```python
from build123d import *

# Parameters (mm, degrees)
F0_R      = 12.5
F1_DEPTH  = 76
F2_W      = 38
F2_H      = 46
F3_DEPTH  = 177
F5_DEPTH  = 67
F6_DEPTH  = 65
F7_W      = 51.9999994738
F7_H      = 11
F8_DEPTH  = 54
F10_DEPTH = 64


with BuildPart() as f1:
    # F0 (on Front) → F1 (new body)
    with BuildSketch(Plane.XZ):
        Polygon((-120, -10.9966229647), (0, -10.9966229647), (0, 7.0033770353), (-56, 7.0033770353), (-56, 61.0033770353), (-120, 61.0033770353), align=None)
        with Locations((-88, 25.0033770353)):
            Circle(F0_R, mode=Mode.SUBTRACT)
    extrude(amount=-F1_DEPTH)

    # F2 (on face) → F3 (cut)
    with BuildSketch(Plane.XY.offset(61.0033770353)):
        with Locations((-88, 36)):
            Rectangle(F2_W, F2_H)
    extrude(amount=-F3_DEPTH, mode=Mode.SUBTRACT)

    # F4 (on face) → F5 (cut)
    with BuildSketch(Plane.XY.offset(7.0033770353)):
        with BuildLine():
            ThreePointArc((-36.0197160629, 75.9483659138), (-10.4386975125, 64.1605543748), (0, 38))
            Line((0, 38), (0, 76))
            Line((0, 76), (-36.0197160629, 75.9483659138))
        make_face()
    extrude(amount=-F5_DEPTH, mode=Mode.SUBTRACT)

    # F4 (on face) → F6 (cut)
    with BuildSketch(Plane.XY.offset(7.0033770353)):
        with BuildLine():
            ThreePointArc((-36.0197160629, 75.9483659138), (-10.4386975125, 64.1605543748), (0, 38))
            Line((0, 38), (0, 76))
            Line((0, 76), (-36.0197160629, 75.9483659138))
        make_face()
        with BuildLine():
            ThreePointArc((0, 38), (-10.3625564741, 11.9198980955), (-35.7985113343, 0.0638240244))
            Line((-35.7985113343, 0.0638240244), (0, 0))
            Line((0, 0), (0, 38))
        make_face()
    extrude(amount=-F6_DEPTH, mode=Mode.SUBTRACT)

    # F7 (on face) → F8 (join)
    with BuildSketch(Plane.XY.offset(7.0033770353)):
        with Locations((-30.0000002631, 32.5063240244)):
            Rectangle(F7_W, F7_H)
        with Locations((-30.0000002631, 43.5063240244)):
            Rectangle(F7_W, F7_H)
    extrude(amount=F8_DEPTH)

    # F9 (on face) → F10 (cut)
    with BuildSketch(Plane.XZ.offset(-27.0063240244)):
        Polygon((-56, 61.0033770353), (-4.0000005262, 7.0033770353), (-4.0000005262, 61.0033770353), align=None)
    extrude(amount=-F10_DEPTH, mode=Mode.SUBTRACT)


solid = f1.part
```
The model under review builds one solid part; all positions refer to its coordinate system, in mm. A direction names the side the tool comes from. Give positions to 0.01 mm unless a question says otherwise; leave off trailing zeros. Loops run counter-clockwise (first coordinate to the right, second up) from the corner with the lowest first, then second, coordinate; pieces in that order, holes last. Notation, with made-up numbers: (30, 37) - (46, 37) arc R26 cw to (46, 68) - close; hole circle Ø7 at (33, 27). An arc over 180 degrees is marked (long way). Answer as a JSON object with one key per item and string values.
Q1. Add section B-B on y = 17.5. State the section outline as (x, z) points.
Worked out:
{"outline": "(-120, -11) - (-107, -11) - (-107, 61) - (-120, 61) - close; (-69, -11) - (-6, -11) - (-6, 7) - (-56, 7) - (-56, 61) - (-69, 61) - close"}
Q2. For faces 4 (the flat face through (-56, 62, 34)), 5 (the flat face through (-69, 36, 26)), 6 (the flat face through (-56, 13, 34)), list the 3-axis set-ups (+Z, -Z, +X, -X, +Y, -Y) from which the entire face can be reached by the end or side of a thin tool; tool diameter is ignored.
Worked out:
{"face 4": "+Z, +X, +Y", "face 5": "+Z, -Z", "face 6": "+Z, +X, -Y"}
Q3. Add section D-D on z = 56.5. State the section outline as (x, y) points.
Worked out:
{"outline": "(-120, 0) - (-56, 0) - (-56, 27.01) - (-51.66, 27.01) - (-51.66, 49.01) - (-56, 49.01) - (-56, 76) - (-120, 76) - close; hole (-107, 13) - (-69, 13) - (-69, 59) - (-107, 59) - close"}
Q4. Add section C-C on x = -104. State the section outline as (y, z) points, plus the area to 3 significant figures.
Worked out:
{"outline": "(0, -11) - (13, -11) - (13, 61) - (0, 61) - close; (59, -11) - (76, -11) - (76, 61) - (59, 61) - close", "area": "2,160 mm^2"}
Q5. Insertion check: pin 1 (8 mm diameter, centred on x = -48.5, z = 40, fed in from +Y); pin 2 (2 mm diameter, centred on y = 45.5, z = 47.5, fed in from +X); pin 3 (3 mm diameter, centred on x = -32.5, y = 49, fed in from +Z). Each pin has a flat end and moves straight along its axis. Give the tip position at first contact, or say it passes through.
Worked out:
{"pin 1": "stops at y = 49.01", "pin 2": "stops at x = -42.03", "pin 3": "stops at z = 38.16"}
Q6. Mouldability with a two-part tool opening along Z and no side actions: class faces 1 (the flat face through (-30.36, 37.85, 34.38)), 2 (the flat face through (-74, 76, 18)), 3 (the cylindrical face through (-76.45, 6.41, 20.22)) as +Z half, -Z half, draft (parallel to the pull), parting line (faces both ways), or undercut.
Worked out:
{"face 1": "+Z half", "face 2": "draft", "face 3": "undercut"}
Q7. Add section A-A on x = -88. State the section outline as (y, z) points, plus the area to 3 significant figures.
Worked out:
{"outline": "(0, -11) - (13, -11) - (13, 12.5) - (0, 12.5) - close; (0, 37.5) - (13, 37.5) - (13, 61) - (0, 61) - close; (59, -11) - (76, -11) - (76, 12.5) - (59, 12.5) - close; (59, 37.5) - (76, 37.5) - (76, 61) - (59, 61) - close", "area": "1,410 mm^2"}
Q8. To check wall thickness, follow line 1 along Y through (x, z) = (-96.5, 45.5); line 2 along X through (y, z) = (17, 44); line 3 along Z through (x, y) = (-88, 65). State the ranges of each line that lie inside material, in increasing order.
Worked out:
{"line 1": "y = 0 to 13, 59 to 76", "line 2": "x = -120 to -107, -69 to -56", "line 3": "z = -11 to 12.5, 37.5 to 61"}
